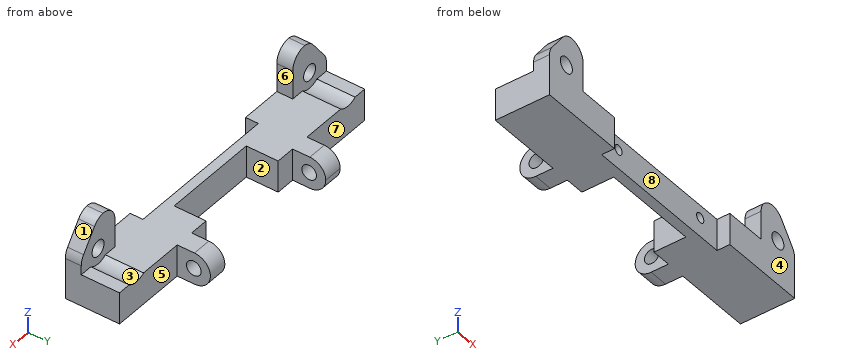
from build123d import *

# Parameters (mm, degrees)
SKETCH1_W           = 51
SKETCH1_H           = 5
BOSS_EXTRUDE1_DEPTH = 8.5
SKETCH2_W           = 15
SKETCH2_H           = 5
CUT_EXTRUDE1_DEPTH  = 5
SKETCH3_W           = 24
SKETCH3_H           = 5
CUT_EXTRUDE2_DEPTH  = 2
SKETCH4_W           = 7
SKETCH4_H           = 2.5
BOSS_EXTRUDE2_DEPTH = 7
SKETCH5_W           = 3
SKETCH5_H           = 5
BOSS_EXTRUDE3_DEPTH = 5.2
SKETCH6_R           = 1.25
CUT_EXTRUDE3_DEPTH  = 30.42685848
SKETCH7_R           = 0.75
CUT_EXTRUDE4_DEPTH  = 5
SKETCH8_R           = 1.15
CUT_EXTRUDE5_DEPTH  = 43.413912812
SKETCH9_R           = 2.5
CUT_EXTRUDE6_DEPTH  = 6
FILLET1_R           = 2.5
CUT_EXTRUDE7_DEPTH  = 30.42685848
FILLET2_R           = 2.5


with BuildPart() as part:
    # Sketch1 → Boss-Extrude1 (new body)
    with BuildSketch(Plane(origin=(0, 0, 0), x_dir=(1, 0, 0), z_dir=(0, 1, 0))):
        Rectangle(SKETCH1_W, SKETCH1_H)
    extrude(amount=BOSS_EXTRUDE1_DEPTH)

    # Sketch2 → Cut-Extrude1 (cut)
    with BuildSketch(Plane(origin=(0, 8.5, 0), x_dir=(1, 0, 0), z_dir=(0, 1, 0))):
        Rectangle(SKETCH2_W, SKETCH2_H)
    extrude(amount=-CUT_EXTRUDE1_DEPTH, mode=Mode.SUBTRACT)

    # Sketch3 → Cut-Extrude2 (cut)
    with BuildSketch(Plane.XZ):
        Rectangle(SKETCH3_W, SKETCH3_H)
    extrude(amount=-CUT_EXTRUDE2_DEPTH, mode=Mode.SUBTRACT)

    # Sketch4 → Boss-Extrude2 (add)
    with BuildSketch(Plane.XY.offset(2.5)):
        with Locations((-22, 1.25)):
            Rectangle(SKETCH4_W, SKETCH4_H)
        with Locations((22, 1.25)):
            Rectangle(SKETCH4_W, SKETCH4_H)
    extrude(amount=BOSS_EXTRUDE2_DEPTH)

    # Sketch5 → Boss-Extrude3 (add)
    with BuildSketch(Plane(origin=(0, 8.5, 0), x_dir=(1, 0, 0), z_dir=(0, 1, 0))):
        with Locations((-12, 0)):
            Rectangle(SKETCH5_W, SKETCH5_H)
        with Locations((12, 0)):
            Rectangle(SKETCH5_W, SKETCH5_H)
    extrude(amount=BOSS_EXTRUDE3_DEPTH)

    # Sketch6 → Cut-Extrude3 (cut, through all)
    with BuildSketch(Plane(origin=(0, 2.5, 0), x_dir=(1, 0, 0), z_dir=(0, 1, 0))):
        with Locations(Location((-22, -4.5, 0), (0, 0, 270))):
            Circle(SKETCH6_R)
        with Locations(Location((22, -4.5, 0), (0, 0, 270))):
            Circle(SKETCH6_R)
    extrude(amount=-CUT_EXTRUDE3_DEPTH, mode=Mode.SUBTRACT)

    # Sketch7 → Cut-Extrude4 (cut)
    with BuildSketch(Plane.XZ.offset(-2)):
        with Locations(Location((-8.5, 0.5, 0), (0, 0, 270))):
            Circle(SKETCH7_R)
        with Locations(Location((8.5, 0.5, 0), (0, 0, 270))):
            Circle(SKETCH7_R)
    extrude(amount=-CUT_EXTRUDE4_DEPTH, mode=Mode.SUBTRACT)

    # Sketch8 → Cut-Extrude5 (cut, through all)
    with BuildSketch(Plane.ZY.offset(13.5)):
        with Locations((0, 11.1)):
            Circle(SKETCH8_R)
    extrude(amount=-CUT_EXTRUDE5_DEPTH, mode=Mode.SUBTRACT)

    # Sketch9 → Cut-Extrude6 (cut)
    with BuildSketch(Plane(origin=(0, 8.5, 0), x_dir=(1, 0, 0), z_dir=(0, 1, 0))):
        with Locations((-22, -4.5)):
            Circle(SKETCH9_R)
        with Locations((22, -4.5)):
            Circle(SKETCH9_R)
    extrude(amount=-CUT_EXTRUDE6_DEPTH, mode=Mode.SUBTRACT)

    # Fillet1
    # the kernel refuses this fillet: 2.5 mm, written as the material it takes off along each edge
    with BuildSketch(Plane(origin=(-25.5, -6.25, 9.5), x_dir=(0, 0, -1), z_dir=(0, 1, 0)), Plane(origin=(-18.5, 8.75, 9.5), x_dir=(0, 0, -1), z_dir=(0, -1, 0))) as fillet1_piece_1:
        with BuildLine():
            CenterArc((FILLET1_R, -FILLET1_R), FILLET1_R, 90, 90)
            Line((0, -FILLET1_R), (0, 0))
            Line((0, 0), (FILLET1_R, 0))
        make_face()
    extrude(amount=15, mode=Mode.SUBTRACT)
    with BuildSketch(Plane(origin=(18.5, 8.75, 9.5), x_dir=(0, 0, -1), z_dir=(0, -1, 0)), Plane(origin=(25.5, -6.25, 9.5), x_dir=(0, 0, -1), z_dir=(0, 1, 0))) as fillet1_piece_2:
        with BuildLine():
            CenterArc((FILLET1_R, FILLET1_R), FILLET1_R, 180, 90)
            Line((0, FILLET1_R), (0, 0))
            Line((0, 0), (FILLET1_R, 0))
        make_face()
    extrude(amount=15, mode=Mode.SUBTRACT)
    with BuildSketch(Plane(origin=(-4.25, 13.7, -2.5), x_dir=(0, 0, 1), z_dir=(-1, 0, 0)), Plane(origin=(19.75, 13.7, 2.5), x_dir=(0, -1, 0), z_dir=(-1, 0, 0))) as fillet1_piece_3:
        with BuildLine():
            CenterArc((FILLET1_R, -FILLET1_R), FILLET1_R, 90, 90)
            Line((0, -FILLET1_R), (0, 0))
            Line((0, 0), (FILLET1_R, 0))
        make_face()
    extrude(amount=15.5, mode=Mode.SUBTRACT)
    with BuildSketch(Plane(origin=(-19.75, 13.7, 2.5), x_dir=(0, -1, 0), z_dir=(1, 0, 0)), Plane(origin=(4.25, 13.7, -2.5), x_dir=(0, 0, 1), z_dir=(1, 0, 0))) as fillet1_piece_4:
        with BuildLine():
            CenterArc((FILLET1_R, FILLET1_R), FILLET1_R, 180, 90)
            Line((0, FILLET1_R), (0, 0))
            Line((0, 0), (FILLET1_R, 0))
        make_face()
    extrude(amount=15.5, mode=Mode.SUBTRACT)

    # Sketch10 → Cut-Extrude7 (cut, through all)
    with BuildSketch(Plane(origin=(0, 2.5, 0), x_dir=(1, 0, 0), z_dir=(0, 1, 0))):
        Polygon((-25.5, -4.75), (-22, -9.5), (-25.5, -9.5), align=None)
        Polygon((25.5, -4.75), (25.5, -9.5), (22, -9.5), align=None)
    extrude(amount=-CUT_EXTRUDE7_DEPTH, mode=Mode.SUBTRACT)

    # Fillet2
    # the kernel refuses this fillet: 2.5 mm, written as the material it takes off along each edge
    with BuildSketch(Plane(origin=(25.5, 4.553949751, 4.75), x_dir=(-0.5931990380498499, 0, 0.8050558373533682), z_dir=(0, -1, 0)), Plane(origin=(-25.5, 4.553949751, 4.75), x_dir=(0, 0, -1), z_dir=(0, -1, 0))) as fillet2_piece_1:
        with BuildLine():
            CenterArc((FILLET2_R * 0.328631960172, FILLET2_R), FILLET2_R, 233.615648184, 36.384351816)
            Line((-FILLET2_R * 0.264567077878, FILLET2_R * 0.194944162647), (-FILLET2_R * 0.276431058639, FILLET2_R * 0.1788430459))
            Line((-FILLET2_R * 0.276431058639, FILLET2_R * 0.1788430459), (-FILLET2_R * 0.00657263920345, -FILLET2_R * 0.02))
            Line((-FILLET2_R * 0.00657263920345, -FILLET2_R * 0.02), (FILLET2_R * 0.328631960172, -FILLET2_R * 0.02))
            Line((FILLET2_R * 0.328631960172, -FILLET2_R * 0.02), (FILLET2_R * 0.328631960172, 0))
        make_face()
    extrude(amount=6.607899502, mode=Mode.SUBTRACT)
    with BuildSketch(Plane(origin=(22, 5.611268046, 9.5), x_dir=(-1, 0, 0), z_dir=(0, -1, 0))) as fillet2_piece_2:
        with BuildLine():
            CenterArc((1.274399108, 2.484895396), FILLET2_R, 216.384351816, 47.314187929)
            Line((-0.738240485, 1.001897801), (-0.778493277, 0.972237849))
            Line((-0.778493277, 0.972237849), (-0.040252792, -0.029659952))
            Line((-0.040252792, -0.029659952), (0, -0.05))
            ThreePointArc((0, -0.05), (0.5, -0.05), (0.994512018, -0.049697908))
            Line((0.994512018, -0.049697908), (1, 0))
        make_face()
    extrude(amount=8.722536093, mode=Mode.SUBTRACT)
    with BuildSketch(Plane(origin=(-22, 5.611268046, 9.5), x_dir=(-0.5931990380498491, 0, -0.8050558373533688), z_dir=(0, -1, 0))) as fillet2_piece_3:
        with BuildLine():
            CenterArc((1.244507219, 2.5), FILLET2_R, 222.685812071, 47.314187929)
            Line((-0.593199038, 0.805055837), (-0.629953163, 0.771156954))
            ThreePointArc((-0.629953163, 0.771156954), (-0.336852311, 0.372867967), (-0.040252792, -0.029659952))
            Line((-0.040252792, -0.029659952), (0, -0.05))
            Line((0, -0.05), (1.244507219, -0.05))
            Line((1.244507219, -0.05), (1.244507219, 0))
        make_face()
    extrude(amount=8.722536093, mode=Mode.SUBTRACT)


solid = part.part
Geometry check sheet. Reference: the model listing, model coordinates, mm. Face numbers are marked on the shaded views. A direction names the side the tool comes from. Round coordinates to 2 decimals unless told otherwise and drop trailing zeros. Loops run counter-clockwise (first coordinate to the right, second up) from the corner with the lowest first, then second, coordinate; pieces in that order, holes last. Notation, with made-up numbers: (-24, 21) - (5, 21) arc R22 ccw to (5, 34) - close; hole circle Ø7 at (86.25, 78.25). An arc over 180 degrees is marked (long way). One line per question, with ' | ' between items. Start each with the question number.
1. Cross-section at B-B on x = -8.5. Record the cut outline in (y, z), then the cut area to 3 significant figures.
2. Cross-section at A-A on y = 1. Record the cut outline in (x, z), then the cut area to 3 significant figures.
3. Tool access check on the marked faces 5, 6, 7 and 8. Record the directions out of +Z, -Z, +X, -X, +Y, -Y that give a thin tool (end or side, any length) a straight path to the whole face; none if there is none.
4. Scan lines: line 1 (X direction, y = 6, z = 0.5); line 2 (Y direction, x = 11.4, z = 0); line 3 (X direction, y = 4, z = -1.25). Record each from-to range of solid material in increasing order. Write a range as [from, to].
5. Cross-section at D-D on z = 4.5. Record the cut outline in (x, y), then the cut area to 3 significant figures.
6. Cross-section at C-C on x = 22. Record the cut outline in (y, z).
7. Draft check along X on the marked faces 1, 2, 3 and 4. Enter one of: released by +X, released by -X, zero draft, split by the parting line, or undercut.
8. Depth check by flat-ended pin: pin 1 (3 mm diameter, centred on x = 22, z = 4.5, fed in from +Y); pin 2 (1.5 mm diameter, centred on y = 12, z = -0.5, fed in from -X); pin 3 (0.6 mm diameter, centred on x = -24.5, y = 5, fed in from +Z). Enter the tip coordinate at first touch or a pass-through.
Taken from the geometry:
1) outline: (2, -2.5) - (8.5, -2.5) - (8.5, 2.5) - (2, 2.5) - (2, 1.25) - (7, 1.25) - (7, -0.25) - (2, -0.25) - close | area: 25.0 mm²
2) outline: (-25.5, -2.5) - (-12, -2.5) - (-12, 2.5) - (-18.5, 2.5) - (-18.5, 7) arc R2.5 ccw to (-21, 9.5) arc R2.5 ccw to (-22.74, 8.5) - (-25.01, 5.41) arc R2.5 ccw to (-25.5, 3.93) - close; (12, -2.5) - (25.5, -2.5) - (25.5, 3.93) arc R2.5 ccw to (25.01, 5.41) - (22.74, 8.5) arc R2.5 ccw to (21, 9.5) arc R2.5 ccw to (18.5, 7) - (18.5, 2.5) - (12, 2.5) - close; hole circle Ø2.5 at (-22, 4.5); hole circle Ø2.5 at (22, 4.5) | area: 203 mm²
3) face 5: +Z, -Z, +X, +Y | face 6: +Z, +Y, -Y | face 7: +Z, -Z, -X, +Y | face 8: +Z, -Z, -Y
4) line 1: [-25.5, -9.25], [-7.75, -7.5], [7.5, 7.75], [9.25, 25.5] | line 2: [2, 9.95], [12.25, 13.7] | line 3: [-25.5, -7.5], [7.5, 25.5]
5) outline: (-25.43, 0) - (-23.25, 0) - (-23.25, 2.5) - (-25.43, 2.5) - close; (-20.75, 0) - (-18.5, 0) - (-18.5, 2.5) - (-20.75, 2.5) - close; (18.5, 0) - (20.75, 0) - (20.75, 2.5) - (18.5, 2.5) - close; (23.25, 0) - (25.43, 0) - (25.43, 2.5) - (23.25, 2.5) - close | area: 22.2 mm²
6) outline: (0, -2.5) - (8.5, -2.5) - (8.5, 2) - (2.5, 2) - (2.5, 3.25) - (0, 3.25) - close; (0, 5.75) - (2.5, 5.75) - (2.5, 9.17) - (0, 9.17) - close
7) face 1: released by +X | face 2: undercut | face 3: undercut | face 4: zero draft
8) pin 1: y = 2.5 | pin 2: x = -13.5 | pin 3: z = 2.5
